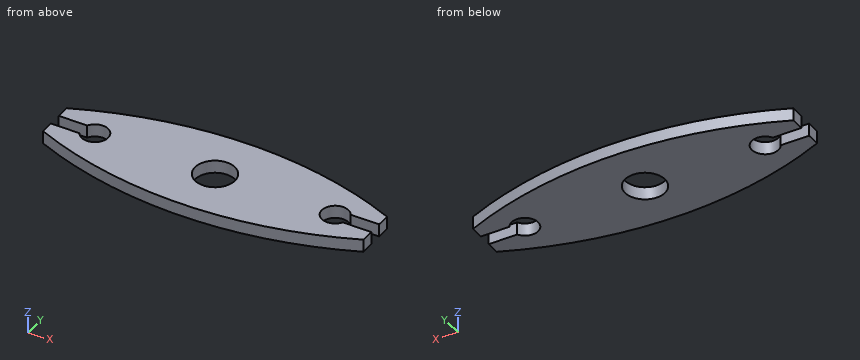
Autodesk Fusion 360 part; units mm, degrees
sketch "Sketch1" plane through (0, 0, 0) normal (0, 0, 1) x (1, 0, 0)
  line L0 (0, 0) -> (304.8, 0) construction
  line L1 (304.8, 0) -> (304.8, 101.6) construction
  line L2 (304.8, 101.6) -> (0, 101.6) construction
  line L3 (0, 101.6) -> (0, 0) construction
  circle A0 centre (152.4, 50.8) radius 19.05
  line L4 (0, 50.8) -> (304.8, 50.8) construction
  line L5 (27.1015, 57.15) -> (0, 57.15)
  line L6 (27.1015, 44.45) -> (0, 44.45)
  line L7 (304.8, 57.15) -> (277.6985, 57.15)
  line L8 (277.6985, 44.45) -> (304.8, 44.45)
  line L9 (0, 69.85) -> (0, 57.15)
  line L10 (0, 44.45) -> (0, 31.75)
  line L11 (304.8, 69.85) -> (304.8, 57.15)
  line L12 (304.8, 44.45) -> (304.8, 31.75)
  arc A1 (27.1015, 44.45) -> (27.1015, 57.15) centre (38.1, 50.8) ccw
  arc A2 (277.6985, 57.15) -> (277.6985, 44.45) centre (266.7, 50.8) ccw
  arc A3 (304.8, 69.85) -> (0, 69.85) centre (152.4, -280.035) ccw
  line L13 (0, 44.45) -> (304.8, 44.45) construction
  line L14 (0, 57.15) -> (304.8, 57.15) construction
  arc A4 (0, 31.75) -> (304.8, 31.75) centre (152.4, 381.635) ccw
  dimension "d1" = 304.8
  dimension "d2" = 101.6
  dimension "d3" = 38.1
  dimension "d5" = 152.4
  dimension "d6" = 25.4
  dimension "d7" = 25.4
  dimension "d8" = 38.1
  dimension "d9" = 38.1
  dimension "d12" = 6.35
  dimension "d13" = 6.35
  dimension "d14" = 12.7
  dimension "d18" = 12.7
extrude "Extrude1" add sketch "Sketch1" along normal blind 12.1412
sketch "Sketch2" plane through (0, 0, 12.1412) normal (0, 0, 1) x (-1, 0, 0)
  circle A0 centre (-152.4, -50.8) radius 19.05
  line L0 (-277.6985, -57.15) -> (-304.8, -57.15)
  line L1 (-304.8, -57.15) -> (-304.8, -69.85)
  arc A1 (-304.8, -69.85) -> (0, -69.85) centre (-152.4, 280.035) ccw
  line L2 (0, -69.85) -> (0, -57.15)
  line L3 (0, -57.15) -> (-27.1015, -57.15)
  line L4 (-27.1015, -44.45) -> (0, -44.45)
  line L5 (0, -44.45) -> (0, -31.75)
  arc A2 (0, -31.75) -> (-304.8, -31.75) centre (-152.4, -381.635) ccw
  line L6 (-304.8, -31.75) -> (-304.8, -44.45)
  line L7 (-304.8, -44.45) -> (-277.6985, -44.45)
  line L8 (-89.0222, -74.9883) -> (-89.0222, -26.3401) construction
  line L9 (-89.0222, -26.3401) -> (-108.0722, -26.3401) construction
  line L10 (-108.0722, -26.3401) -> (-108.0722, -74.9883) construction
  line L11 (-108.0722, -74.9883) -> (-89.0222, -74.9883) construction
  line L12 (-152.4, -101.6) -> (-152.4, 0) construction
  arc A3 (-277.6985, -57.15) -> (-277.6985, -44.45) centre (-266.7, -50.8) ccw
  arc A4 (-27.1015, -44.45) -> (-27.1015, -57.15) centre (-38.1, -50.8) ccw
Check sheet for the modelled part. Datum: model origin and axes. Units: mm. Round coordinates to 2 decimals unless told otherwise and drop trailing zeros. Order: outer loops, then holes, each group sorted by start corner. A loop starts at its lowest first (then second) coordinate and runs counter-clockwise, first axis right, second up.
1) Section check B-B (x = 152.4). Record the boundary of the cut face in (y, z), and give its area (3 significant figures).
2) Scan lines: line 1 (Y direction, x = 152.4, z = 4.25); line 2 (X direction, y = 60, z = 11); line 3 (X direction, y = 67, z = 2). Record each from-to range of solid material in increasing order.
3) Section check D-D (y = 16). Record the boundary of the cut face in (x, z), and give its area (3 significant figures).
4) Section check A-A (y = 50.8). Record the boundary of the cut face in (x, z).
5) Go/stop test with flat-tipped pins: pin 1 Ø2 at (x, z) = (74, 6) entering from +Y; pin 2 Ø1 at (x, z) = (58, 6.5) entering from +Y; pin 3 Ø23 at (x, y) = (266.7, 50.8) entering from -Z; pin 4 Ø6 at (x, z) = (95, 4.5) entering from +Y. Record where each tip stops, or that it passes through.
Result:
1. outline: (0, 0) - (31.75, 0) - (31.75, 12.14) - (0, 12.14) - close; (69.85, 0) - (101.6, 0) - (101.6, 12.14) - (69.85, 12.14) - close
1. area: 771 mm2
2. line 1: y = 0 to 31.75, 69.85 to 101.6
2. line 2: x = 0 to 29.35, 46.85 to 135.72, 169.08 to 257.95, 275.45 to 304.8
2. line 3: x = 0 to 142.38, 162.42 to 304.8
3. outline: (43.06, 0) - (261.74, 0) - (261.74, 12.14) - (43.06, 12.14) - close
3. area: 2,660 mm2
4. outline: (50.8, 0) - (133.35, 0) - (133.35, 12.14) - (50.8, 12.14) - close; (171.45, 0) - (254, 0) - (254, 12.14) - (171.45, 12.14) - close
5. pin 1: stops at y = 93.67
5. pin 2: stops at y = 89.87
5. pin 3: passes through
5. pin 4: stops at y = 97.7
